CAD build for the part. Positions are in the model's coordinates, mm. A direction names the side the tool comes from. Coordinates: 2 decimals unless noted, no trailing zeros. Loops run counter-clockwise (first coordinate to the right, second up) from the corner with the lowest first, then second, coordinate; pieces in that order, holes last.
1) Saw through at B-B, the plane x = 15.5. Write the cut outline in (y, z), and give its area (3 significant figures).
2) Which spindle directions (+Z, -Z, +X, -X, +Y, -Y) get a long thin tool onto all of the face, cutting with end or side? Do faces 4 (the flat face through (-38.1, 454, 1)), 5 (the flat face through (-1, 454, -38.1)), 6 (the flat face through (38.1, 454, 1)). Say none if no direction does.
3) Two-plate mould, pull along Y, no slides. Class faces 1 (the flat face through (-1, 685.8, -1)), 2 (the flat face through (-5, 0, -5)), 3 (the flat face through (114.3, 151, 2)): +Y half, -Y half, draft (parallel to the pull), parting line (faces both ways), or undercut.
4) Saw through at A-A, the plane z = -28. Write the cut outline in (x, y), and give its area (3 significant figures).
5) Pin check, flat tips, straight feed: pin 1 Ø23 at (y, z) = (403, -2.5) entering from +X; pin 2 Ø5 at (y, z) = (84, 105.5) entering from -X; pin 3 Ø23 at (x, y) = (-10.5, 374.5) entering from -Z. Stop position of each tip, or through.
6) Saw through at C-C, the plane y = 632.5. Write the cut outline in (x, z), and give its area (3 significant figures).
7) Saw through at D-D, the plane x = -99. Write the cut outline in (y, z).
8) Wall check: line 1 along Y through (x, z) = (-249, 298.5); line 2 along X through (y, z) = (148, 7); line 3 along Y through (x, z) = (94, 87). Give the ranges that are in metal, low to high.
```python
from build123d import *

# Parameters (mm, degrees)
SKETCH1_W           = 76.2
SKETCH1_H           = 76.2
BOSS_EXTRUDE1_DEPTH = 685.8
SKETCH1_3_W         = 228.6
SKETCH1_3_H         = 228.6
SKETCH1_3_W_2       = 76.2
SKETCH1_3_H_2       = 76.2
BOSS_EXTRUDE2_DEPTH = 228.6
SKETCH1_4_W         = 685.8
SKETCH1_4_H         = 685.8
SKETCH1_4_W_2       = 228.6
SKETCH1_4_H_2       = 228.6
BOSS_EXTRUDE3_DEPTH = 76.2


with BuildPart() as part:
    # Sketch1 → Boss-Extrude1 (new body)
    with BuildSketch(Plane(origin=(0, 0, 0), x_dir=(1, 0, 0), z_dir=(0, 1, 0))):
        Rectangle(SKETCH1_W, SKETCH1_H)
    extrude(amount=BOSS_EXTRUDE1_DEPTH)

    # Sketch1<3> → Boss-Extrude2 (add)
    with BuildSketch(Plane(origin=(0, 0, 0), x_dir=(1, 0, 0), z_dir=(0, 1, 0))):
        Rectangle(SKETCH1_3_W, SKETCH1_3_H)
        Rectangle(SKETCH1_3_W_2, SKETCH1_3_H_2, mode=Mode.SUBTRACT)
    extrude(amount=BOSS_EXTRUDE2_DEPTH)

    # Sketch1<4> → Boss-Extrude3 (add)
    with BuildSketch(Plane(origin=(0, 0, 0), x_dir=(1, 0, 0), z_dir=(0, 1, 0))):
        Rectangle(SKETCH1_4_W, SKETCH1_4_H)
        Rectangle(SKETCH1_4_W_2, SKETCH1_4_H_2, mode=Mode.SUBTRACT)
    extrude(amount=BOSS_EXTRUDE3_DEPTH)


solid = part.part
```
Data:
1. outline: (0, -342.9) - (76.2, -342.9) - (76.2, -114.3) - (228.6, -114.3) - (228.6, -38.1) - (685.8, -38.1) - (685.8, 38.1) - (228.6, 38.1) - (228.6, 114.3) - (76.2, 114.3) - (76.2, 342.9) - (0, 342.9) - close
1. area: 122,000 mm2
2. face 4: +Z, -Z, -X, +Y
2. face 5: -Z, +X, -X, +Y
2. face 6: +Z, -Z, +X, +Y
3. face 1: +Y half
3. face 2: -Y half
3. face 3: draft
4. outline: (-342.9, 0) - (342.9, 0) - (342.9, 76.2) - (114.3, 76.2) - (114.3, 228.6) - (38.1, 228.6) - (38.1, 685.8) - (-38.1, 685.8) - (-38.1, 228.6) - (-114.3, 228.6) - (-114.3, 76.2) - (-342.9, 76.2) - close
4. area: 122,000 mm2
5. pin 1: stops at x = 38.1
5. pin 2: stops at x = -114.3
5. pin 3: stops at z = -38.1
6. outline: (-38.1, -38.1) - (38.1, -38.1) - (38.1, 38.1) - (-38.1, 38.1) - close
6. area: 5,810 mm2
7. outline: (0, -342.9) - (76.2, -342.9) - (76.2, -114.3) - (228.6, -114.3) - (228.6, 114.3) - (76.2, 114.3) - (76.2, 342.9) - (0, 342.9) - close
8. line 1: y = 0 to 76.2
8. line 2: x = -114.3 to 114.3
8. line 3: y = 0 to 228.6
